```python
from build123d import *

# Parameters (mm, degrees)
SKETCH_R      = 20.5
PAD_DEPTH     = 3
SKETCH001_R   = 4
SKETCH001_R_2 = 1.75
POCKET_DEPTH  = 3.001


with BuildPart() as part:
    # Sketch → Pad (new body)
    with BuildSketch(Plane.XY):
        with Locations((40, 40)):
            Circle(SKETCH_R)
    extrude(amount=PAD_DEPTH)

    # Sketch001 → Pocket (cut, through all)
    with BuildSketch(Plane.XY):
        with Locations((40, 40)):
            Circle(SKETCH001_R)
        with Locations((28.155961, 28.155961)):
            Circle(SKETCH001_R_2)
        with Locations((51.844039, 28.155961)):
            Circle(SKETCH001_R_2)
        with Locations((51.844039, 51.844039)):
            Circle(SKETCH001_R_2)
        with Locations((28.155961, 51.844039)):
            Circle(SKETCH001_R_2)
    extrude(amount=POCKET_DEPTH, mode=Mode.SUBTRACT)


solid = part.part
```
The listing builds one solid part. Answer for the finished solid, in the listing's coordinates (mm). Give positions to 0.01 mm unless a question says otherwise; leave off trailing zeros. Loops run counter-clockwise (first coordinate to the right, second up) from the corner with the lowest first, then second, coordinate; pieces in that order, holes last. Notation, with made-up numbers: (11.25, 29.5) - (56.25, 29.5) arc R26 cw to (56.25, 60.5) - close; hole circle Ø5 at (-27.75, -33.5). An arc over 180 degrees is marked (long way). Return JSON: item names as keys, results as strings. Group by question number.
1. Find section A-A (y = 40). Write down the section's boundary in (x, z), then the cut area to 3 significant figures.
2. Determine the mould class of faces 1 (the flat face through (44.3, 40.3, 0)), 2 (the cylindrical face through (29.773, 27.486, 1.479)), 3 (the cylindrical face through (59.553, 46.158, 1.479)) for opening direction X: pulls with the +X half, pulls with the -X half, needs draft (parallel to the pull), parting line crosses it, or undercut.
3. Find section C-C (x = 51). Write down the section's boundary in (y, z).
4. Given pin 1 Ø1 at (x, z) = (51, 1) entering from +Y; pin 2 Ø1.5 at (y, z) = (50.5, 0.5) entering from -X, each flat-ended and moving along its own axis, determine where each tip first touches the part or whether it passes through.
5. Find section D-D (z = 2.4). Write down the section's boundary in (x, y), then the cut area to 3 significant figures.
6. Straight lines are drawn through the part: line 1 (X direction, y = 50.5, z = 2.3); line 2 (X direction, y = 28.5, z = 0.25); line 3 (X direction, y = 42.5, z = 1.85). For each, find the intervals that lie inside material, in ascending order. Write a range as [from, to].
Verdict:
{
 "1": {"outline": "(19.5, 0) - (36, 0) - (36, 3) - (19.5, 3) - close; (44, 0) - (60.5, 0) - (60.5, 3) - (44, 3) - close", "area": "99.0 mm^2"},
 "2": {"face 1": "needs draft", "face 2": "undercut", "face 3": "parting line crosses it"},
 "3": {"outline": "(22.7, 0) - (26.62, 0) - (26.62, 3) - (22.7, 3) - close; (29.69, 0) - (50.31, 0) - (50.31, 3) - (29.69, 3) - close; (53.38, 0) - (57.3, 0) - (57.3, 3) - (53.38, 3) - close"},
 "4": {"pin 1": "stops at y = 57.61", "pin 2": "stops at x = 21.97"},
 "5": {"outline": "circle Ø41 at (40, 40); hole circle Ø3.5 at (28.16, 28.16); hole circle Ø3.5 at (28.16, 51.84); hole circle Ø8 at (40, 40); hole circle Ø3.5 at (51.84, 28.16); hole circle Ø3.5 at (51.84, 51.84)", "area": "1,230 mm^2"},
 "6": {"line 1": "x = [22.39, 27.04], [29.28, 50.72], [52.96, 57.61]", "line 2": "x = [23.03, 26.44], [29.87, 50.13], [53.56, 56.97]", "line 3": "x = [19.65, 36.88], [43.12, 60.35]"}
}
